Design review of the part shown in the three views and the two pictorial views. Dimensions are in mm from the part's minimum x, y and z. A direction names the side the tool comes from. Round coordinates to 2 decimals unless told otherwise and drop trailing zeros. Loops run counter-clockwise (first coordinate to the right, second up) from the corner with the lowest first, then second, coordinate; pieces in that order, holes last. Notation, with made-up numbers: (72, 7.25) -> (86, 7.25) arc R33 cw to (86, 38.25) -> close; hole circle Ø11 at (-35.75, -29.5). An arc over 180 degrees is marked (long way). Return JSON: item names as keys, results as strings. Group by question number.
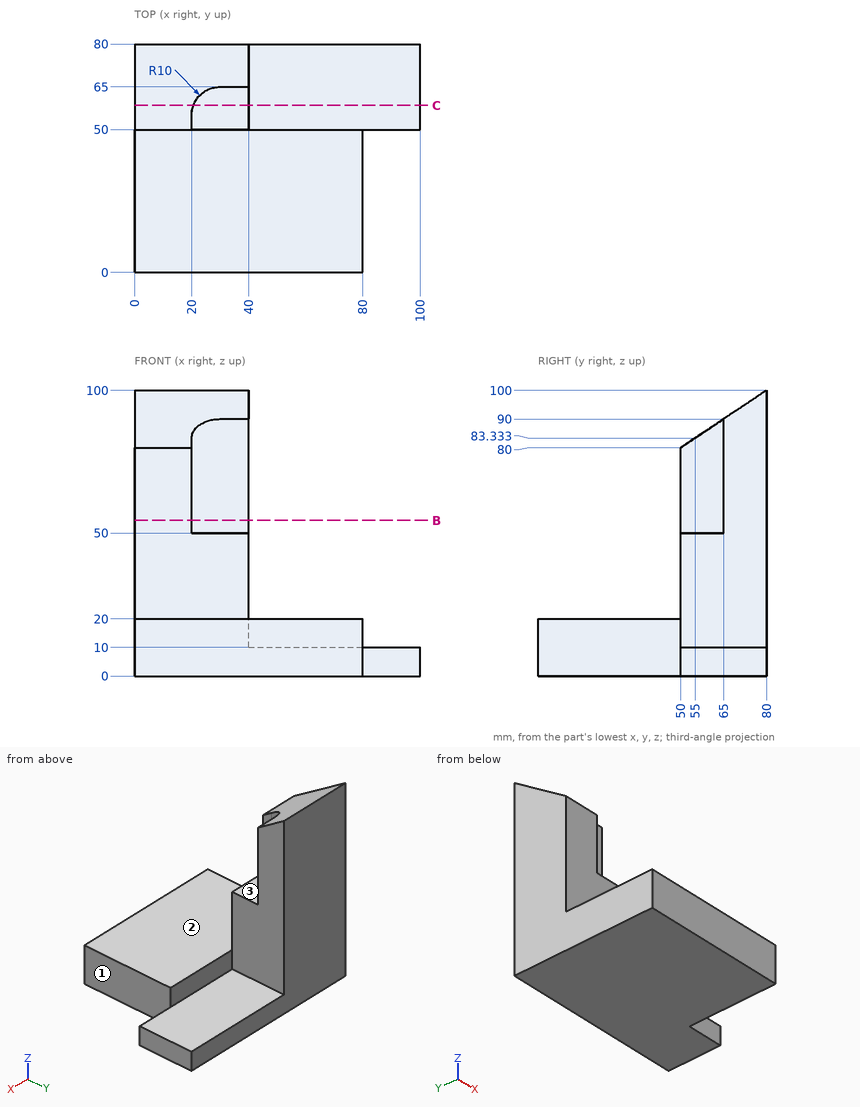
1. Wall thickness on line 1 (Y direction, x = 24.5, z = 40); line 2 (Z direction, x = 81.5, y = 61.5); line 3 (Z direction, x = 65, y = 30.5): over which ranges is each line inside the solid? List them lowest first.
2. For P1, Ø4.5, axis at x = 29.5, y = 55.5, coming from the +Z side; P2, Ø5, axis at x = 19, z = 66.5, coming from the -Y side; P3, Ø4, axis at y = 72, z = 81.5, coming from the -X side; P4, Ø6, axis at x = 54, y = 60, coming from the +Z side, all flat-tipped, find the tip position at first contact; note any pin that passes through.
3. We need section B-B, the plane z = 54.5. Write out the cut boundary in (x, y).
4. We need section C-C, the plane y = 58.5. Write out the cut boundary in (x, z), then the cut area to 3 significant figures.
5. Tool access review of the marked faces 1, 2 and 3: name each direction out of +Z, -Z, +X, -X, +Y, -Y from which nothing blocks a thin tool from reaching the whole face with its end or side.
Check sheet entries:
{
 "1": {"line 1": "y = 50 to 80", "line 2": "z = 0 to 10", "line 3": "z = 0 to 20"},
 "2": {"P1": "stops at z = 50", "P2": "stops at y = 50", "P3": "stops at x = 0", "P4": "stops at z = 10"},
 "3": {"outline": "(0, 50) -> (20, 50) -> (20, 55) arc R10 cw to (30, 65) -> (40, 65) -> (40, 80) -> (0, 80) -> close"},
 "4": {"outline": "(0, 0) -> (100, 0) -> (100, 10) -> (40, 10) -> (40, 50) -> (20.63, 50) -> (20.63, 85.67) -> (0, 85.67) -> close", "area": "3,340 mm²"},
 "5": {"face 1": "+Z, -Z, +X, -Y", "face 2": "+Z, +X, -X, -Y", "face 3": "+Z, +X, -Y"}
}
